The model under review builds one solid part; all positions refer to its coordinate system, in mm. Coordinates: 2 decimals unless noted, no trailing zeros. Loops run counter-clockwise (first coordinate to the right, second up) from the corner with the lowest first, then second, coordinate; pieces in that order, holes last. Notation, with made-up numbers: M 36,31.25 L 65,31.25 A21 ccw 65,69.25 Z; hole C -13.5,43 d5. An arc over 180 degrees is marked long. One line per item, written item: value.
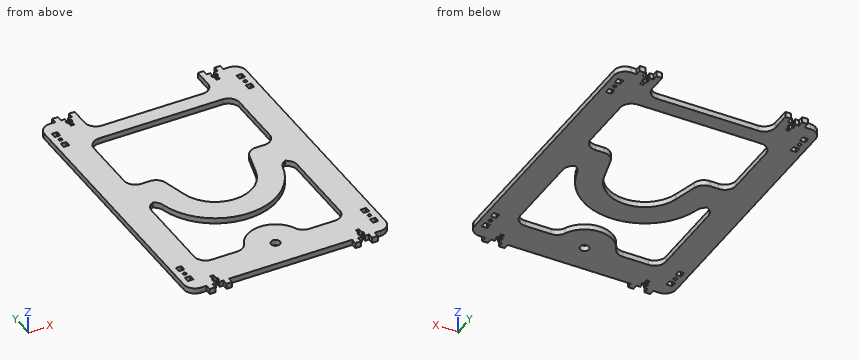
```python
from build123d import *

# Parameters (mm, degrees)
SKETCH1_W           = 5
SKETCH1_H           = 5
SKETCH1_R           = 1.5
SKETCH1_R_2         = 4
BOSS_EXTRUDE1_DEPTH = 5
FILLET1_R           = 10


with BuildPart() as part:
    # Sketch1 → Boss-Extrude1 (new body)
    with BuildSketch(Plane.XY):
        Polygon((-75, 125), (-90, 125), (-90, -125), (-75, -125), (-75, -130), (-70, -130), (-70, -125), (-66.5, -125), (-66.5, -122), (-67.6, -122), (-67.6, -119.7), (-66.5, -119.7), (-66.5, -115), (-63.5, -115), (-63.5, -119.7), (-62.4, -119.7), (-62.4, -122), (-63.5, -122), (-63.5, -125), (-60, -125), (-60, -130), (-55, -130), (-55, -125), (55, -125), (55, -130), (60, -130), (60, -125), (63.5, -125), (63.5, -122), (62.4, -122), (62.4, -119.7), (63.5, -119.7), (63.5, -115), (66.5, -115), (66.5, -119.7), (67.6, -119.7), (67.6, -122), (66.5, -122), (66.5, -125), (70, -125), (70, -130), (75, -130), (75, -125), (90, -125), (90, 125), (75, 125), (75, 130), (70, 130), (70, 125), (66.5, 125), (66.5, 122), (67.6, 122), (67.6, 119.7), (66.5, 119.7), (66.5, 115), (63.5, 115), (63.5, 119.7), (62.4, 119.7), (62.4, 122), (63.5, 122), (63.5, 125), (60, 125), (60, 130), (55, 130), (55, 103.598832104), (-55, 103.598832104), (-55, 130), (-60, 130), (-60, 125), (-63.5, 125), (-63.5, 122), (-62.4, 122), (-62.4, 119.7), (-63.5, 119.7), (-63.5, 115), (-66.5, 115), (-66.5, 119.7), (-67.6, 119.7), (-67.6, 122), (-66.5, 122), (-66.5, 125), (-70, 125), (-70, 130), (-75, 130), align=None)
        with Locations((-82.5, -110)):
            Rectangle(SKETCH1_W, SKETCH1_H, mode=Mode.SUBTRACT)
        with Locations((-82.5, -102.5)):
            Circle(SKETCH1_R, mode=Mode.SUBTRACT)
        with Locations((-82.5, -95)):
            Rectangle(SKETCH1_W, SKETCH1_H, mode=Mode.SUBTRACT)
        with Locations((0, -100)):
            Circle(SKETCH1_R_2, mode=Mode.SUBTRACT)
        with Locations((82.5, -110)):
            Rectangle(SKETCH1_W, SKETCH1_H, mode=Mode.SUBTRACT)
        with Locations((82.5, -102.5)):
            Circle(SKETCH1_R, mode=Mode.SUBTRACT)
        with Locations((82.5, -95)):
            Rectangle(SKETCH1_W, SKETCH1_H, mode=Mode.SUBTRACT)
        with BuildLine():
            Line((-65, -5.570672252), (-54.717160111, -5.570672252))
            ThreePointArc((-54.717160111, -5.570672252), (0, -55), (54.717160111, -5.570672252))
            Line((54.717160111, -5.570672252), (65, -5.570672252))
            Line((65, -5.570672252), (65, -95.958016924))
            Line((65, -95.958016924), (24.671083738, -95.958016924))
            ThreePointArc((24.671083738, -95.958016924), (0, -75), (-24.671083738, -95.958016924))
            Line((-24.671083738, -95.958016924), (-65, -95.958016924))
            Line((-65, -95.958016924), (-65, -5.570672252))
        make_face(mode=Mode.SUBTRACT)
        with Locations((-82.5, 95)):
            Rectangle(SKETCH1_W, SKETCH1_H, mode=Mode.SUBTRACT)
        with Locations((-82.5, 102.5)):
            Circle(SKETCH1_R, mode=Mode.SUBTRACT)
        with Locations((-82.5, 110)):
            Rectangle(SKETCH1_W, SKETCH1_H, mode=Mode.SUBTRACT)
        with BuildLine():
            ThreePointArc((31.875552268, -8.541028488), (0, -33), (-31.875552268, -8.541028488))
            Line((-31.875552268, -8.541028488), (-39.523097802, 20))
            Line((-39.523097802, 20), (-65, 20))
            Line((-65, 20), (-65, 89.539551807))
            Line((-65, 89.539551807), (65, 89.539551807))
            Line((65, 89.539551807), (65, 20))
            Line((65, 20), (39.523097802, 20))
            Line((39.523097802, 20), (31.875552268, -8.541028488))
        make_face(mode=Mode.SUBTRACT)
        with Locations((82.5, 95)):
            Rectangle(SKETCH1_W, SKETCH1_H, mode=Mode.SUBTRACT)
        with Locations((82.5, 102.5)):
            Circle(SKETCH1_R, mode=Mode.SUBTRACT)
        with Locations((82.5, 110)):
            Rectangle(SKETCH1_W, SKETCH1_H, mode=Mode.SUBTRACT)
    extrude(amount=BOSS_EXTRUDE1_DEPTH)

    # Fillet1
    # the kernel refuses this fillet: 10 mm, written as the material it adds along each edge
    with BuildSketch(Plane(origin=(-55, 103.598832104, 0), x_dir=(1, 0, 0), z_dir=(0, 0, 1)), Plane(origin=(55, 103.598832104, 0), x_dir=(0, 1, 0), z_dir=(0, 0, 1)), Plane(origin=(-65, -95.958016924, 0), x_dir=(1, 0, 0), z_dir=(0, 0, 1)), Plane(origin=(65, -95.958016924, 0), x_dir=(0, 1, 0), z_dir=(0, 0, 1)), Plane(origin=(65, -5.570672252, 0), x_dir=(-1, 0, 0), z_dir=(0, 0, 1)), Plane(origin=(-65, -5.570672252, 0), x_dir=(0, -1, 0), z_dir=(0, 0, 1)), Plane(origin=(65, 89.539551807, 0), x_dir=(-1, 0, 0), z_dir=(0, 0, 1)), Plane(origin=(-65, 89.539551807, 0), x_dir=(0, -1, 0), z_dir=(0, 0, 1)), Plane(origin=(65, 20, 0), x_dir=(0, 1, 0), z_dir=(0, 0, 1)), Plane(origin=(-65, 20, 0), x_dir=(1, 0, 0), z_dir=(0, 0, 1))) as fillet1_piece_1:
        with BuildLine():
            CenterArc((FILLET1_R, FILLET1_R), FILLET1_R, 180, 90)
            Line((0, FILLET1_R), (0, 0))
            Line((0, 0), (FILLET1_R, 0))
        make_face()
    extrude(amount=5)
    with BuildSketch(Plane(origin=(24.671083738, -95.958016924, 0), x_dir=(1, 0, 0), z_dir=(0, 0, 1))) as fillet1_piece_2:
        with BuildLine():
            CenterArc((7.388590485, 10), FILLET1_R, 203.653187484, 66.346812516)
            ThreePointArc((-1.771316436, 5.988004835), (-0.697963006, 3.049524687), (0, 0))
            Line((0, 0), (7.388590485, 0))
        make_face()
    extrude(amount=5)
    with BuildSketch(Plane(origin=(-24.671083738, -95.958016924, 0), x_dir=(-1, 0, 0), z_dir=(0, 0, 1))) as fillet1_piece_3:
        with BuildLine():
            CenterArc((7.388590485, -10), FILLET1_R, 90, 66.346812516)
            ThreePointArc((-1.771316436, -5.988004835), (-0.697963006, -3.049524687), (0, 0))
            Line((0, 0), (7.388590485, 0))
        make_face()
    extrude(amount=5)
    with BuildSketch(Plane(origin=(54.717160111, -5.570672252, 0), x_dir=(-0.17083790481511615, -0.9852991476086749, 0), z_dir=(0, 0, 1))) as fillet1_piece_4:
        with BuildLine():
            CenterArc((8.419606625, 9.975355126), FILLET1_R, 189.836540175, 76.140088059)
            Line((-1.433384851, 8.266976078), (0, 0))
            ThreePointArc((0, 0), (3.85898637, 0.135546807), (7.717972739, 0))
        make_face()
    extrude(amount=5)
    with BuildSketch(Plane(origin=(-54.717160111, -5.570672252, 0), x_dir=(-1, 0, 0), z_dir=(0, 0, 1))) as fillet1_piece_5:
        with BuildLine():
            CenterArc((8.390320948, 10), FILLET1_R, 193.859911941, 76.140088059)
            ThreePointArc((-1.318522292, 7.604511961), (-0.525706993, 3.825412513), (0, 0))
            Line((0, 0), (8.390320948, 0))
        make_face()
    extrude(amount=5)
    # the kernel refuses this fillet: 10 mm, written as the material it takes off along each edge
    with BuildSketch(Plane(origin=(-90, -125, -25), x_dir=(0, 1, 0), z_dir=(0, 0, 1)), Plane(origin=(90, -125, -25), x_dir=(-1, 0, 0), z_dir=(0, 0, 1)), Plane(origin=(-90, 125, -25), x_dir=(1, 0, 0), z_dir=(0, 0, 1)), Plane(origin=(90, 125, -25), x_dir=(0, -1, 0), z_dir=(0, 0, 1))) as fillet1_2_piece_1:
        with BuildLine():
            CenterArc((FILLET1_R, -FILLET1_R), FILLET1_R, 90, 90)
            Line((0, -FILLET1_R), (0, 0))
            Line((0, 0), (FILLET1_R, 0))
        make_face()
    extrude(amount=55, mode=Mode.SUBTRACT)
    with BuildSketch(Plane(origin=(39.523097802, 20, -19.183174699), x_dir=(1, 0, 0), z_dir=(0, 0, 1)), Plane(origin=(-39.523097802, 20, -19.183174699), x_dir=(0.2588190451025106, -0.9659258262890711, 0), z_dir=(0, 0, 1))) as fillet1_2_piece_2:
        with BuildLine():
            CenterArc((FILLET1_R * 0.767326987979, -FILLET1_R), FILLET1_R, 90, 75)
            Line((-FILLET1_R * 0.19859883831, -FILLET1_R * 0.741180954897), (0, 0))
            Line((0, 0), (FILLET1_R * 0.767326987979, 0))
        make_face()
    extrude(amount=43.366349399, mode=Mode.SUBTRACT)


solid = part.part
```
(1) To check wall thickness, follow L1, parallel to X at y = 102.5, z = 1.85; L2, parallel to X at y = 57.5, z = 3.1; L3, parallel to X at y = -102.5, z = 2.5. State the ranges of each line that lie inside material, in increasing order. Write a range as [from, to].
Checks:
L1: [-90, -84], [-81, 81], [84, 90]
L2: [-90, -65], [65, 90]
L3: [-90, -84], [-81, -3.12], [3.12, 81], [84, 90]
(2) Add section A-A on x = 0. State the section outline as (y, z) points.
Checks:
outline: M -125,0 L -104,0 L -104,5 L -125,5 Z; M -96,0 L -75,0 L -75,5 L -96,5 Z; M -55,0 L -33,0 L -33,5 L -55,5 Z; M 89.54,0 L 103.6,0 L 103.6,5 L 89.54,5 Z
(3) Add section C-C on z = 2.35. State how many separate pieces and enclosed holes the cut face has, then the cut area to 3 significant figures.
Checks:
separate pieces: 1
enclosed holes: 15
area: 23,500 mm^2
(4) Insertion check: pin 1 Ø1.5 at (y, z) = (123.5, 2.5) entering from +X; pin 2 Ø1.5 at (x, z) = (-78, 2) entering from -Y; pin 3 Ø2.5 at (y, z) = (-123.5, 3.5) entering from +X. Each pin has a flat end and moves straight along its axis. Give the tip position at first contact, or say it passes through.
Checks:
pin 1: x = 86.32
pin 2: y = -125
pin 3: x = 86.89
(5) Add section B-B on y = 71. State the section outline as (x, z) points, then the cut area to 3 significant figures.
Checks:
outline: M -90,0 L -65,0 L -65,5 L -90,5 Z; M 65,0 L 90,0 L 90,5 L 65,5 Z
area: 250 mm^2
